The listing builds one solid part. Answer for the finished solid, in the listing's coordinates (mm). A direction names the side the tool comes from. Give positions to 0.01 mm unless a question says otherwise; leave off trailing zeros. Write each loop counter-clockwise with the first axis right and the second up, starting at its lowest first coordinate (ties: lowest second). Pieces come first, ordered by that corner, then holes. Notation, with made-up numbers: M 54.25,-34 L 91.25,-34 A31 ccw 91.25,-5 Z; hole C -23,-5.75 d10. An arc over 180 degrees is marked long. Return JSON: item names as keys, results as strings.
from build123d import *

# Parameters (mm, degrees)
BOSS_EXTRUDE1_DEPTH = 22
SKETCH3_R           = 3.75
BOSS_EXTRUDE2_DEPTH = 15
SKETCH7_R           = 1.75
CUT_EXTRUDE3_DEPTH  = 6
CUT_EXTRUDE4_DEPTH  = 3


with BuildPart() as part:
    # Sketch2 → Boss-Extrude1 (new body)
    with BuildSketch(Plane(origin=(0, 0, 0), x_dir=(1, 0, 0), z_dir=(0, 1, 0))):
        Polygon((23, 0), (-9, 0), (-9, -6), (13, -6), (13, -16), (23, -16), align=None)
    extrude(amount=BOSS_EXTRUDE1_DEPTH)

    # Sketch3 → Boss-Extrude2 (add)
    with BuildSketch(Plane.XY.offset(6)):
        with Locations(Location((-3, 11, 0), (0, 0, 180))):
            Circle(SKETCH3_R)
    extrude(amount=BOSS_EXTRUDE2_DEPTH)

    # Sketch7 → Cut-Extrude3 (cut)
    with BuildSketch(Plane.XY.offset(16)):
        with Locations((18, 16.5)):
            Circle(SKETCH7_R)
        with Locations((18, 5.5)):
            Circle(SKETCH7_R)
    extrude(amount=-CUT_EXTRUDE3_DEPTH, mode=Mode.SUBTRACT)

    # Sketch8 → Cut-Extrude4 (cut)
    with BuildSketch(Plane.XY.offset(16)):
        Polygon((21.25, 14.623611625), (21.25, 18.376388375), (18, 20.25277675), (14.75, 18.376388375), (14.75, 14.623611625), (18, 12.74722325), align=None)
        Polygon((21.25, 3.623611625), (21.25, 7.376388375), (18, 9.25277675), (14.75, 7.376388375), (14.75, 3.623611625), (18, 1.74722325), align=None)
    extrude(amount=-CUT_EXTRUDE4_DEPTH, mode=Mode.SUBTRACT)


solid = part.part
Item 1: Given pin 1 Ø3 at (x, y) = (18, 5.5) entering from +Z; pin 2 Ø7 at (x, y) = (18, 16) entering from +Z; pin 3 Ø5 at (y, z) = (15.5, 10.5) entering from -X, each flat-ended and moving along its own axis, determine where each tip first touches the part or whether it passes through.
Geometry results:
{"pin 1": "stops at z = 10", "pin 2": "stops at z = 16", "pin 3": "stops at x = -6.17"}
Item 2: A cutting plane is placed at A-A, the plane z = 7. Write down the section's boundary in (x, y), plus the area to 3 significant figures.
Geometry results:
{"outline": "C -3,11 d7.5; M 13,0 L 23,0 L 23,22 L 13,22 Z", "area": "264 mm2"}
Item 3: A cutting plane is placed at D-D, the plane z = 17.5. Write down the section's boundary in (x, y).
Geometry results:
{"outline": "C -3,11 d7.5"}
Item 4: A cutting plane is placed at B-B, the plane y = 11. Write down the section's boundary in (x, z).
Geometry results:
{"outline": "M -9,0 L 23,0 L 23,16 L 13,16 L 13,6 L 0.75,6 L 0.75,21 L -6.75,21 L -6.75,6 L -9,6 Z"}
Item 5: Find the intervals of material crossed by line 1 (Y direction, x = 18, z = 11.35); line 2 (Y direction, x = 18, z = 14.25); line 3 (Z direction, x = 22, y = 2.5), in increasing order.
Geometry results:
{"line 1": "y = 0 to 3.75, 7.25 to 14.75, 18.25 to 22", "line 2": "y = 0 to 1.75, 9.25 to 12.75, 20.25 to 22", "line 3": "z = 0 to 16"}
Item 6: A cutting plane is placed at C-C, the plane x = -3. Write down the section's boundary in (y, z).
Geometry results:
{"outline": "M 0,0 L 22,0 L 22,6 L 14.75,6 L 14.75,21 L 7.25,21 L 7.25,6 L 0,6 Z"}
Item 7: Which of the six approach directions +Z, -Z, +X, -X, +Y, -Y give full straight-line access (tool end or side, diameter ignored) to faces 1 (the flat face through (-9, 11, 3)), 2 (the flat face through (16.35, 13.7, 14.52)), 3 (the flat face through (18, 11, 16))?
Geometry results:
{"face 1": "+Z, -Z, -X, +Y, -Y", "face 2": "+Z", "face 3": "+Z, +X, +Y, -Y"}
Item 8: Determine the mould class of faces 4 (the cylindrical face through (-2.512, 7.282, 13.395)), 5 (the flat face through (19.65, 8.3, 14.52)), 6 (the flat face through (19.65, 19.3, 14.52)), 7 (the flat face through (13, 11, 11)) for opening direction Y: +Y half, -Y half, draft (parallel to the pull), parting line (faces both ways), or undercut.
Geometry results:
{"face 4": "parting line", "face 5": "undercut", "face 6": "undercut", "face 7": "draft"}
